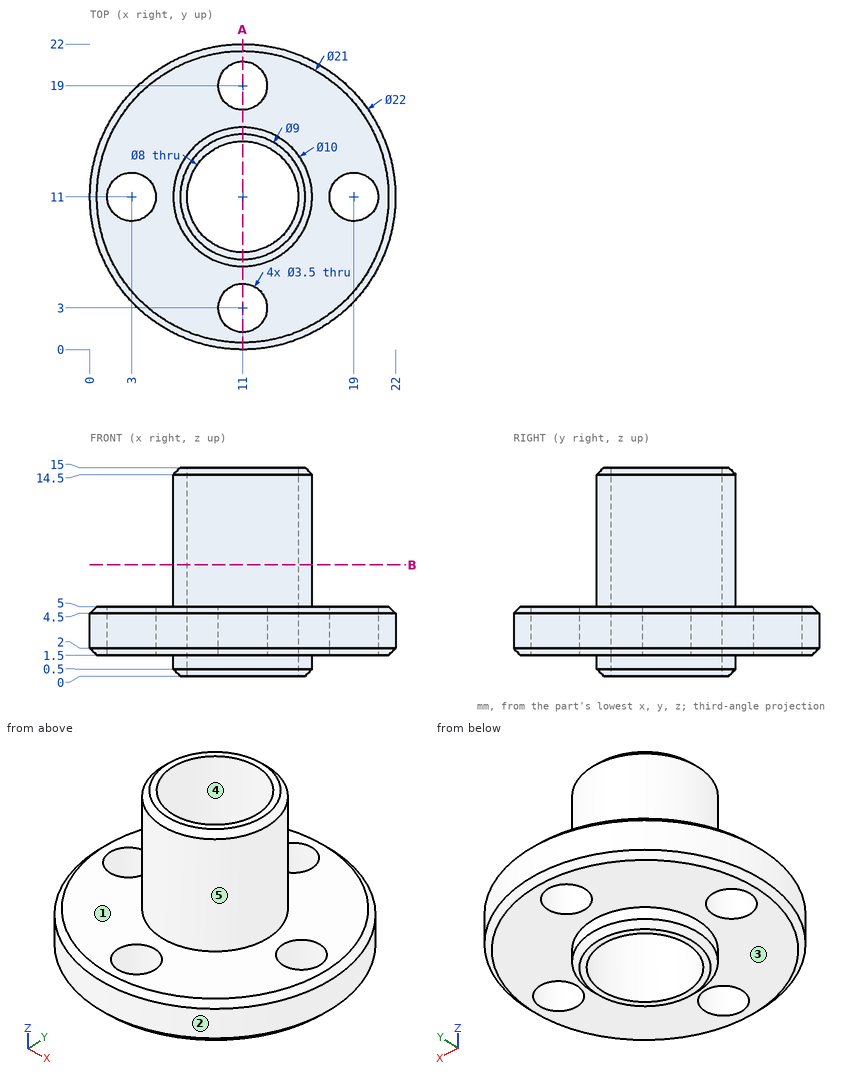
The figure shows three views and two pictorial views of one solid part (mm, origin at its lowest corner). Answer the questions. A direction names the side the tool comes from. Give positions to 0.01 mm unless a question says otherwise; leave off trailing zeros. Order: outer loops, then holes, each group sorted by start corner. A loop starts at its lowest first (then second) coordinate and runs counter-clockwise, first axis right, second up. Notation, with made-up numbers: (48, 22.5) -> (67, 22.5) arc R26 ccw to (67, 47.5) -> close; hole circle Ø1 at (83, -35.75). An arc over 180 degrees is marked (long way). Answer as a JSON object with one key per item and string values. Group by question number.
Item 1: Consider L1, parallel to Y at x = 11, z = 2.75; L2, parallel to X at y = 10.5, z = 4.75; L3, parallel to Y at x = 11, z = 7.5. Determine where each line is inside the solid, lowest interval first. Write a range as from..to.
Item 2: The part is cut by section B-B on z = 8. Write down the section's boundary in (x, y).
Item 3: Flat-ended cylindrical pins translate along their axes: pin 1 (4.5 mm diameter, centred on x = 3, y = 11, fed in from +Z); pin 2 (3 mm diameter, centred on x = 18, y = 7.5, fed in from -Z); pin 3 (8 mm diameter, centred on x = 18.5, z = 6, fed in from -Y). Find the tip coordinate at first contact, or state that the pin passes through.
Item 4: A tool of negligible diameter and unlimited length cuts with its end or side. For the marked faces 1 and 2, from which of +Z, -Z, +X, -X, +Y, -Y can it reach the whole face along a straight path? Write none if from no direction.
Item 5: The part is cut by section A-A on x = 11. Give the number of separate pieces and of enclosed holes in the cut face, and give its area (3 significant figures).
Item 6: Determine the mould class of the marked faces 3, 4 and 5 for opening direction X: pulls with the +X half, pulls with the -X half, needs draft (parallel to the pull), parting line crosses it, or undercut.
Result set:
{
 "1": {"L1": "0..1.25, 4.75..7, 15..17.25, 20.75..22", "L2": "0.26..1.32, 4.68..7.03, 14.97..17.32, 20.68..21.74", "L3": "6..7, 15..16"},
 "2": {"outline": "circle Ø10 at (11, 11); hole circle Ø8 at (11, 11)"},
 "3": {"pin 1": "z = 5", "pin 2": "z = 1.5", "pin 3": "y = 0.67"},
 "4": {"face 1": "+Z", "face 2": "+Z, -Z"},
 "5": {"separate pieces": "4", "enclosed holes": "0", "area": "46.5 mm²"},
 "6": {"face 3": "needs draft", "face 4": "undercut", "face 5": "parting line crosses it"}
}
